```python
from build123d import *

# Parameters (mm, degrees)
SKETCH1_W           = 3870.96
SKETCH1_H           = 22014.18
BOSS_EXTRUDE1_DEPTH = 161.29
SKETCH2_W           = 3870.96
SKETCH2_H           = 17780
BOSS_EXTRUDE2_DEPTH = 161.29
SKETCH3_W           = 3870.96
SKETCH3_H           = 17780
BOSS_EXTRUDE3_DEPTH = 161.29
SKETCH4_W           = 3870.96
SKETCH4_H           = 3709.67
BOSS_EXTRUDE4_DEPTH = 15261.336
SKETCH5_R           = 161.29
CUT_EXTRUDE1_DEPTH  = 12848.844
SKETCH7_R           = 1282.7
CUT_EXTRUDE2_DEPTH  = 21138.454907405
SCALE1_SCALE        = 0.039370079


with BuildPart() as part:
    # Sketch1 → Boss-Extrude1 (new body)
    with BuildSketch(Plane.XY):
        Rectangle(SKETCH1_W, SKETCH1_H)
    extrude(amount=BOSS_EXTRUDE1_DEPTH)

    # Sketch2 → Boss-Extrude2 (add)
    with BuildSketch(Plane(origin=(0, 11007.09, 0), x_dir=(1, 0, 0), z_dir=(0, 1, 0))):
        with Locations((0, 8890)):
            Rectangle(SKETCH2_W, SKETCH2_H)
    extrude(amount=-BOSS_EXTRUDE2_DEPTH)

    # Sketch3 → Boss-Extrude3 (add)
    with BuildSketch(Plane(origin=(0, 4415.536, 0), x_dir=(1, 0, 0), z_dir=(0, 1, 0))):
        with Locations((0, 8890)):
            Rectangle(SKETCH3_W, SKETCH3_H)
    extrude(amount=-BOSS_EXTRUDE3_DEPTH)

    # Sketch4 → Boss-Extrude4 (add)
    with BuildSketch(Plane.XZ.offset(-4254.246)):
        with Locations((0, -1786.014661267)):
            Rectangle(SKETCH4_W, SKETCH4_H)
    extrude(amount=BOSS_EXTRUDE4_DEPTH)

    # Sketch5 → Cut-Extrude1 (cut)
    with BuildSketch(Plane(origin=(0, 11007.09, 0), x_dir=(1, 0, 0), z_dir=(0, 1, 0))):
        with Locations(Location((0, 17258.03, 0), (0, 0, 270))):
            Circle(SKETCH5_R)
        with Locations(Location((0, 10161.27, 0), (0, 0, 270))):
            Circle(SKETCH5_R)
    extrude(amount=-CUT_EXTRUDE1_DEPTH, mode=Mode.SUBTRACT)

    # Sketch7 → Cut-Extrude2 (cut, through all)
    with BuildSketch(Plane.XY.offset(161.29)):
        with Locations((0, -9216.39)):
            Circle(SKETCH7_R)
    extrude(amount=-CUT_EXTRUDE2_DEPTH, mode=Mode.SUBTRACT)


with BuildPart() as part_1:
    # Scale1: scaled about (0, -1625.758634815, -2390.119236931)
    add(part.part.scale(SCALE1_SCALE).moved(Location((0, -1561.75238935, -2296.020054375))))


solid = part_1.part
```
Geometry: final body of the model. Coordinates: model frame, mm. A direction names the side the tool comes from. Give positions to 0.01 mm unless a question says otherwise; leave off trailing zeros. Write each loop counter-clockwise with the first axis right and the second up, starting at its lowest first coordinate (ties: lowest second). Pieces come first, ordered by that corner, then holes.
1. Reachability of faces 1 (the flat face through (76.2, -1688, -2357)), 2 (the flat face through (-1, -1260, -2296.02)), 3 (the flat face through (-1, -1394.262, -2722)) from +Z, -Z, +X, -X, +Y, -Y: full face, straight path, thin tool, end or side. Return the list, or none.
2. Draft query along Y for faces 4 (the flat face through (-1, -1690, -2439.361)), 5 (the flat face through (-1, -1134.752, -2651)), 6 (the flat face through (-1, -1128.402, -2648)). Return one class per face: released by +Y, released by -Y, zero draft, split by the parting line, or undercut.
3. Section query B-B, the plane z = -2398.5. Return loops of the section in (x, y).
4. Pin query (flat end, axial travel): P1, Ø5, axis at x = 61, y = -1842.5, coming from the -Z side; P2, Ø7.5, axis at x = 0, z = -2975.47, coming from the -Y side; P3, Ø2, axis at x = 8, z = -2575, coming from the -Y side. Return the tip coordinate at first contact, or that it passes through.
5. Section query C-C, the plane y = -1264.5. Return loops of the section in (x, z), then the cut area to 3 significant figures.
6. Section query D-D, the plane x = -18. Return loops of the section in (y, z).
7. Line query: probe 1 along Y at (x, z) = (-1.5, -2443.5); probe 2 along Y at (x, z) = (6.5, -2354.5); probe 3 along Z at (x, y) = (-37, -1354). Output: solid intervals per line, ascending.
8. Section query A-A, the plane x = 34.5. Return loops of the section in (y, z).
Computed:
1. face 1: +Z, -Z, +X, +Y, -Y
1. face 2: -Z, +X, -X
1. face 3: -Z, +X, -X, -Y
2. face 4: zero draft
2. face 5: undercut
2. face 6: released by +Y
3. outline: (-76.2, -1995.1) - (76.2, -1995.1) - (76.2, -1387.91) - (-76.2, -1387.91) - close; (-76.2, -1134.75) - (76.2, -1134.75) - (76.2, -1128.4) - (-76.2, -1128.4) - close; hole circle Ø101 at (0, -1924.6)
4. P1: stops at z = -2439.36
4. P2: passes through
4. P3: stops at y = -1394.26
5. outline: (-76.2, -2296.02) - (76.2, -2296.02) - (76.2, -2289.67) - (-76.2, -2289.67) - close
5. area: 968 mm2
6. outline: (-1995.1, -2439.36) - (-1971.79, -2439.36) - (-1971.79, -2289.67) - (-1995.1, -2289.67) - close; (-1877.42, -2439.36) - (-1394.26, -2439.36) - (-1394.26, -2996.02) - (-1387.91, -2996.02) - (-1387.91, -2296.02) - (-1134.75, -2296.02) - (-1134.75, -2996.02) - (-1128.4, -2996.02) - (-1128.4, -2289.67) - (-1877.42, -2289.67) - close
7. probe 1: y = -1394.26 to -1387.91, -1134.75 to -1128.4
7. probe 2: y = -1995.1 to -1974.68, -1874.52 to -1387.91, -1134.75 to -1128.4
7. probe 3: z = -2296.02 to -2289.67
8. outline: (-1995.1, -2439.36) - (-1961.48, -2439.36) - (-1961.48, -2289.67) - (-1995.1, -2289.67) - close; (-1887.72, -2439.36) - (-1394.26, -2439.36) - (-1394.26, -2996.02) - (-1387.91, -2996.02) - (-1387.91, -2296.02) - (-1134.75, -2296.02) - (-1134.75, -2996.02) - (-1128.4, -2996.02) - (-1128.4, -2289.67) - (-1887.72, -2289.67) - close
